Build history of the part. All positions in model axes, mm. A direction names the side the tool comes from. Round coordinates to 2 decimals unless told otherwise and drop trailing zeros. Write each loop counter-clockwise with the first axis right and the second up, starting at its lowest first coordinate (ties: lowest second). Pieces come first, ordered by that corner, then holes. Notation, with made-up numbers: M 33,73 L 91,73 A17 cw 91,104 Z; hole C -22.5,69.25 d1. An arc over 180 degrees is marked long. One line per item, written item: value. Start each with the question number.
Autodesk Inventor part; units mm, degrees
ref_plane "YZ Plane" through (0, 0, 0) normal (1, 0, 0) x (0, 1, 0)
ref_plane "XZ Plane" through (0, 0, 0) normal (0, 1, 0) x (-1, 0, 0)
ref_plane "XY Plane" through (0, 0, 0) normal (0, 0, 1) x (1, 0, 0)
sketch "Sketch1" plane through (0, 0, 0) normal (0, 0, 1) x (1, 0, 0)
  line L0 (-70, -10) -> (70, -10)
  line L1 (70, -10) -> (70, 10)
  line L2 (70, 10) -> (-70, 10)
  line L3 (-70, 10) -> (-70, -10)
  point P0 (0, 0)
  dimension "width" = 140
  dimension "d1" = 70
  dimension "d2" = 20
  dimension "d3" = 10
extrude "Extrusion1" add sketch "Sketch1" along normal blind 5
sketch "Sketch4" plane through (-70, -10, 0) normal (0, -1, 0) x (1, 0, 0)
  line L0 (0, 0) -> (140, 0)
  line L1 (0, 5) -> (140, 5)
  line L2 (0, 0) -> (24.8, 0)
  line L3 (24.8, 0) -> (24.8, 5)
  line L4 (24.8, 5) -> (0, 5)
  line L5 (0, 5) -> (0, 0)
  point P0 (70, 0)
  dimension "d28" = 24.8
extrude "Extrusion4" add sketch "Sketch4" along normal blind 5
mirror "Mirror1" about plane through (0, 0, 0) normal (1, 0, 0) of "Extrusion4"
properties part number "EBF_003.1-front-plate_cup-holder"
Item 1: Two-plate mould, pull along X, no slides. Class faces 1 (the flat face through (-1, -2, 0)), 2 (the flat face through (45.2, -12, 3)), 3 (the flat face through (-70, -2, 2)), 4 (the flat face through (70, -2, 2)): pulls with the +X half, pulls with the -X half, needs draft (parallel to the pull), parting line crosses it, or undercut.
Item 2: Which spindle directions (+Z, -Z, +X, -X, +Y, -Y) get a long thin tool onto all of the face, cutting with end or side? Do faces 5 (the flat face through (-1, -10, 2)), 6 (the flat face through (57, -15, 3)). Say none if no direction does.
Item 3: Drop a flat-ended pin along its axis: pin 1 (1 mm diameter, centred on x = 24.5, z = 3.5, fed in from -Y). Give the stop position or say it passes through.
Item 4: Cut at C-C, the plane x = -33. Write the cut outline in (y, z), plus the area to 3 significant figures.
Item 5: Drill centre lines: line 1 (X direction, y = -11, z = 2.8); line 2 (Y direction, x = 24, z = 3.95). Where is each one in solid material? Low to high.
Item 6: Cut at B-B, the plane z = 3.9. Write the cut outline in (x, y).
Item 7: Cut at A-A, the plane y = -12.5. Write the cut outline in (x, z), plus the area to 3 significant figures.
Computed values:
1. face 1: needs draft
1. face 2: undercut
1. face 3: pulls with the -X half
1. face 4: pulls with the +X half
2. face 5: +Z, -Z, -Y
2. face 6: +Z, -Z, +X, -X, -Y
3. pin 1: stops at y = -10
4. outline: M -10,0 L 10,0 L 10,5 L -10,5 Z
4. area: 100 mm2
5. line 1: x = -70 to -45.2, 45.2 to 70
5. line 2: y = -10 to 10
6. outline: M -70,-15 L -45.2,-15 L -45.2,-10 L 45.2,-10 L 45.2,-15 L 70,-15 L 70,10 L -70,10 Z
7. outline: M -70,0 L -45.2,0 L -45.2,5 L -70,5 Z; M 45.2,0 L 70,0 L 70,5 L 45.2,5 Z
7. area: 248 mm2
